```python
from build123d import *

# Parameters (mm, degrees)
BOSS_EXTRUDE1_DEPTH     = 10
SKETCH2_W               = 17.2
SKETCH2_H               = 43
CUT_EXTRUDE1_DEPTH      = 72.414284285
SKETCH3_W               = 90
SKETCH3_H               = 34
SKETCH3_W_2             = 80
SKETCH3_H_2             = 24
BOSS_EXTRUDE3_DEPTH     = 15
SKETCH4_W               = 49.6
SKETCH4_H               = 5
BOSS_EXTRUDE4_DEPTH     = 10
SKETCH5_W               = 15
SKETCH5_H               = 22
BOSS_EXTRUDE5_DEPTH     = 5
SKETCH6_W               = 90
SKETCH6_H               = 77
BOSS_EXTRUDE6_DEPTH     = 15
BOSS_EXTRUDE8_DEPTH     = 39
CHAMFER1_SIZE           = 64
CHAMFER1_SIZE_2         = 3.354097874
CHAMFER2_SIZE           = 64
CHAMFER2_SIZE_2         = 11.405813635
CHAMFER3_SIZE           = 64
CHAMFER3_SIZE_2         = 13.775745352
CUT_EXTRUDE3_DEPTH      = 95.500525601
CUT_EXTRUDE3_DEPTH_BACK = 95.500525601
SKETCH10_W              = 50
SKETCH10_H              = 27
SKETCH15_R              = 8
CUT_EXTRUDE5_DEPTH      = 122.227059686
CUT_EXTRUDE6_DEPTH      = 2.5
SKETCH18_W              = 29.6
SKETCH18_H              = 43
CUT_EXTRUDE7_DEPTH      = 10
CUT_EXTRUDE8_DEPTH      = 15
SKETCH21_W              = 29.6
SKETCH21_H              = 33
BOSS_EXTRUDE10_DEPTH    = 2.5
SKETCH23_W              = 2.05
SKETCH23_H              = 13
BOSS_EXTRUDE11_DEPTH    = 15
SKETCH24_OUTSIDE_W      = 133.046
SKETCH24_OUTSIDE_H      = 133.046
SKETCH24_OUTSIDE_W_2    = 90
SKETCH24_OUTSIDE_H_2    = 72
CUT_EXTRUDE10_DEPTH     = 61.5
SKETCH26_W              = 100
SKETCH26_H              = 100
CUT_EXTRUDE13_DEPTH     = 10


with BuildPart() as part:
    # Sketch1 → Boss-Extrude1 (new body)
    with BuildSketch(Plane(origin=(0, 0, 0), x_dir=(1, 0, 0), z_dir=(0, 1, 0))):
        with BuildLine():
            Line((-35, 50), (35, 50))
            ThreePointArc((35, 50), (45.606601718, 45.606601718), (50, 35))
            Line((50, 35), (50, -35))
            ThreePointArc((50, -35), (45.606601718, -45.606601718), (35, -50))
            Line((35, -50), (-35, -50))
            ThreePointArc((-35, -50), (-45.606601718, -45.606601718), (-50, -35))
            Line((-50, -35), (-50, 35))
            ThreePointArc((-50, 35), (-45.606601718, 45.606601718), (-35, 50))
        make_face()
    extrude(amount=BOSS_EXTRUDE1_DEPTH)

    # Sketch2 → Cut-Extrude1 (cut, through all)
    with BuildSketch(Plane(origin=(0, 10, 0), x_dir=(1, 0, 0), z_dir=(0, 1, 0))):
        with Locations((-33.4, 18.5)):
            Rectangle(SKETCH2_W, SKETCH2_H)
        with Locations((33.4, 18.5)):
            Rectangle(SKETCH2_W, SKETCH2_H)
    extrude(amount=-CUT_EXTRUDE1_DEPTH, mode=Mode.SUBTRACT)

    # Sketch3 → Boss-Extrude3 (add)
    with BuildSketch(Plane(origin=(0, 10, 0), x_dir=(1, 0, 0), z_dir=(0, 1, 0))):
        with Locations((0, -20)):
            Rectangle(SKETCH3_W, SKETCH3_H)
        with Locations((0, -20)):
            Rectangle(SKETCH3_W_2, SKETCH3_H_2, mode=Mode.SUBTRACT)
    extrude(amount=BOSS_EXTRUDE3_DEPTH)

    # Sketch4 → Boss-Extrude4 (add)
    with BuildSketch(Plane(origin=(0, 10, 0), x_dir=(1, 0, 0), z_dir=(0, 1, 0))):
        with Locations((0, 10)):
            Rectangle(SKETCH4_W, SKETCH4_H)
        with Locations((0, 27)):
            Rectangle(SKETCH4_W, SKETCH4_H)
    extrude(amount=BOSS_EXTRUDE4_DEPTH)

    # Sketch5 → Boss-Extrude5 (add)
    with BuildSketch(Plane(origin=(0, 20, 0), x_dir=(1, 0, 0), z_dir=(0, 1, 0))):
        with Locations((-17.3, 18.5)):
            Rectangle(SKETCH5_W, SKETCH5_H)
        with Locations((17.3, 18.5)):
            Rectangle(SKETCH5_W, SKETCH5_H)
    extrude(amount=BOSS_EXTRUDE5_DEPTH)

    # Sketch6 → Boss-Extrude6 (add)
    with BuildSketch(Plane(origin=(0, 10, 0), x_dir=(1, 0, 0), z_dir=(0, 1, 0))):
        with BuildLine():
            Line((-50, 35), (-50, -35))
            ThreePointArc((-50, -35), (-45.606601718, -45.606601718), (-35, -50))
            Line((-35, -50), (35, -50))
            ThreePointArc((35, -50), (45.606601718, -45.606601718), (50, -35))
            Line((50, -35), (50, 35))
            ThreePointArc((50, 35), (45.606601718, 45.606601718), (35, 50))
            Line((35, 50), (-35, 50))
            ThreePointArc((-35, 50), (-45.606601718, 45.606601718), (-50, 35))
        make_face()
        with Locations((0, 1.5)):
            Rectangle(SKETCH6_W, SKETCH6_H, mode=Mode.SUBTRACT)
    extrude(amount=BOSS_EXTRUDE6_DEPTH)

    # Sketch9 → Boss-Extrude8 (add)
    with BuildSketch(Plane(origin=(0, 25, 0), x_dir=(1, 0, 0), z_dir=(0, 1, 0))):
        with BuildLine():
            Line((-50, 35), (-50, -35))
            ThreePointArc((-50, -35), (-45.606601718, -45.606601718), (-35, -50))
            Line((-35, -50), (35, -50))
            ThreePointArc((35, -50), (45.606601718, -45.606601718), (50, -35))
            Line((50, -35), (50, 35))
            ThreePointArc((50, 35), (45.606601718, 45.606601718), (35, 50))
            Line((35, 50), (-35, 50))
            ThreePointArc((-35, 50), (-45.606601718, 45.606601718), (-50, 35))
        make_face()
        with BuildLine():
            Line((-45, 35), (-45, -32))
            Line((-45, -32), (45, -32))
            Line((45, -32), (45, 35))
            ThreePointArc((45, 35), (44.659258263, 37.588190451), (43.660254038, 40))
            Line((43.660254038, 40), (-43.660254038, 40))
            ThreePointArc((-43.660254038, 40), (-44.659258263, 37.588190451), (-45, 35))
        make_face(mode=Mode.SUBTRACT)
    extrude(amount=BOSS_EXTRUDE8_DEPTH)

    # Chamfer1
    # the kernel refuses this chamfer: 64, 3.354097874 mm, written as the material it takes off along each edge
    with BuildSketch(Plane(origin=(-35, 64, 50), x_dir=(0, -0.9999979738662979, 0.002013023422382214), z_dir=(1, 0, 0)), Plane(origin=(50, 64, 35), x_dir=(0.002013023422382214, -0.9999979738662979, 0), z_dir=(0, 0, -1)), Plane(origin=(-50, 64, -35), x_dir=(-0.002013023422382214, -0.9999979738662979, 0), z_dir=(0, 0, 1)), Plane(origin=(35, 64, -50), x_dir=(0, -0.9999979738662979, -0.002013023422382214), z_dir=(-1, 0, 0))) as chamfer1_piece_1:
        Polygon((CHAMFER1_SIZE * 0.999997973866, CHAMFER1_SIZE * 0.00201302342238), (-CHAMFER1_SIZE_2 * 0.00201302342245, CHAMFER1_SIZE_2 * 0.9999979739), (0, 0), align=None)
    extrude(amount=70, mode=Mode.SUBTRACT)
    with BuildSketch(Plane(origin=(35, 64, 35), x_dir=(0, 0, 1), z_dir=(-1, 0, 0))) as chamfer1_piece_2:
        Polygon((15, -CHAMFER1_SIZE), (15 - CHAMFER1_SIZE_2, 0), (15, 0), align=None)
    revolve(axis=Axis((35, 64, 35), (0, 1, 0)), revolution_arc=90, mode=Mode.SUBTRACT)
    with BuildSketch(Plane(origin=(-35, 64, 35), x_dir=(-1, 0, 0), z_dir=(0, 0, -1))) as chamfer1_piece_3:
        Polygon((15, -CHAMFER1_SIZE), (15 - CHAMFER1_SIZE_2, 0), (15, 0), align=None)
    revolve(axis=Axis((-35, 64, 35), (0, 1, 0)), revolution_arc=90, mode=Mode.SUBTRACT)
    with BuildSketch(Plane(origin=(35, 64, -35), x_dir=(1, 0, 0), z_dir=(0, 0, 1))) as chamfer1_piece_4:
        Polygon((15, -CHAMFER1_SIZE), (15 - CHAMFER1_SIZE_2, 0), (15, 0), align=None)
    revolve(axis=Axis((35, 64, -35), (0, 1, 0)), revolution_arc=90, mode=Mode.SUBTRACT)
    with BuildSketch(Plane(origin=(-35, 64, -35), x_dir=(0, 0, -1), z_dir=(1, 0, 0))) as chamfer1_piece_5:
        Polygon((15 - CHAMFER1_SIZE_2, 0), (15, -CHAMFER1_SIZE), (15, 0), align=None)
    revolve(axis=Axis((-35, 64, -35), (0, 1, 0)), revolution_arc=90, mode=Mode.SUBTRACT)

    # Chamfer2
    # the kernel refuses this chamfer: 64, 11.405813635 mm, written as the material it takes off along each edge
    with BuildSketch(Plane(origin=(201.306482971, 64, -46.645902126), x_dir=(0, -0.9982575003065525, -0.05900816114499234), z_dir=(-1, 0, 0))) as chamfer2_piece_1:
        Polygon((CHAMFER2_SIZE * 0.999977671636, CHAMFER2_SIZE * 0.0066825316561), (-CHAMFER2_SIZE_2 * 0.0590081611462, CHAMFER2_SIZE_2 * 0.998257500326), (0, 0), align=None)
    extrude(amount=402.612965942, mode=Mode.SUBTRACT)

    # Chamfer3
    # the kernel refuses this chamfer: 64, 13.775745352 mm, written as the material it takes off along each edge
    with BuildSketch(Plane(origin=(-201.265469314, 64, 46.645902126), x_dir=(0, -0.9981787050157903, 0.06032638604292662), z_dir=(1, 0, 0))) as chamfer3_piece_1:
        Polygon((CHAMFER3_SIZE * 0.999967974892, CHAMFER3_SIZE * 0.00800307379952), (-CHAMFER3_SIZE_2 * 0.060326386045, CHAMFER3_SIZE_2 * 0.99817870505), (0, 0), align=None)
    extrude(amount=402.530938629, mode=Mode.SUBTRACT)

    # Sketch10 → Cut-Extrude3 (cut, two sides: drawn at the far end of the back side and taken through both)
    with BuildSketch(Plane(origin=(0, 1.307501734, 0), x_dir=(0, 0, 1), z_dir=(-1, 0, 0)).offset(-CUT_EXTRUDE3_DEPTH_BACK)):
        with Locations((-22.129843227, 49.192498266)):
            Rectangle(SKETCH10_W, SKETCH10_H)
    extrude(amount=CUT_EXTRUDE3_DEPTH + CUT_EXTRUDE3_DEPTH_BACK, mode=Mode.SUBTRACT)

    # Sketch15 → Cut-Extrude5 (cut, through all)
    with BuildSketch(Plane.XY.offset(-40)):
        with Locations((-12.75, 20.25)):
            Circle(SKETCH15_R)
        with Locations((12.75, 20.25)):
            Circle(SKETCH15_R)
    extrude(amount=-CUT_EXTRUDE5_DEPTH, mode=Mode.SUBTRACT)

    # Sketch17 → Cut-Extrude6 (cut)
    with BuildSketch(Plane(origin=(0, 0, -29.5), x_dir=(-1, 0, 0), z_dir=(0, 0, -1))):
        Polygon((-24.8, 10), (24.8, 10), (24.8, 25), (9.8, 25), (9.8, 20), (-9.8, 20), (-9.8, 25), (-24.8, 25), align=None)
    extrude(amount=-CUT_EXTRUDE6_DEPTH, mode=Mode.SUBTRACT)

    # Sketch18 → Cut-Extrude7 (cut)
    with BuildSketch(Plane.XZ):
        with Locations((0, -18.5)):
            Rectangle(SKETCH18_W, SKETCH18_H)
    extrude(amount=-CUT_EXTRUDE7_DEPTH, mode=Mode.SUBTRACT)

    # Sketch20 → Cut-Extrude8 (cut)
    with BuildSketch(Plane.XZ.offset(-25)):
        with BuildLine():
            Line((-45, -35), (-45, -40))
            Line((-45, -40), (-43.660254038, -40))
            ThreePointArc((-43.660254038, -40), (-44.659258263, -37.588190451), (-45, -35))
        make_face()
        with BuildLine():
            Line((45, -40), (45, -35))
            ThreePointArc((45, -35), (44.659258263, -37.588190451), (43.660254038, -40))
            Line((43.660254038, -40), (45, -40))
        make_face()
    extrude(amount=-CUT_EXTRUDE8_DEPTH, mode=Mode.SUBTRACT)

    # Sketch21 → Boss-Extrude10 (add)
    with BuildSketch(Plane.XZ):
        with Locations((0, -13.5)):
            Rectangle(SKETCH21_W, SKETCH21_H)
    extrude(amount=-BOSS_EXTRUDE10_DEPTH)

    # Sketch23 → Boss-Extrude11 (add)
    with BuildSketch(Plane(origin=(0, 10, 0), x_dir=(1, 0, 0), z_dir=(0, 1, 0))):
        with Locations((-23.775, 33.5)):
            Rectangle(SKETCH23_W, SKETCH23_H)
        with Locations((23.775, 33.5)):
            Rectangle(SKETCH23_W, SKETCH23_H)
    extrude(amount=BOSS_EXTRUDE11_DEPTH)

    # Sketch24 outside → Cut-Extrude10 (cut)
    with BuildSketch(Plane(origin=(0, 64, 0), x_dir=(1, 0, 0), z_dir=(0, 1, 0))):
        Rectangle(SKETCH24_OUTSIDE_W, SKETCH24_OUTSIDE_H)
        with Locations((0, 4)):
            Rectangle(SKETCH24_OUTSIDE_W_2, SKETCH24_OUTSIDE_H_2, mode=Mode.SUBTRACT)
    extrude(amount=-CUT_EXTRUDE10_DEPTH, mode=Mode.SUBTRACT)

    # Sketch26 → Cut-Extrude13 (cut)
    with BuildSketch(Plane.XZ):
        Rectangle(SKETCH26_W, SKETCH26_H)
    extrude(amount=-CUT_EXTRUDE13_DEPTH, mode=Mode.SUBTRACT)


with BuildPart() as body_2:
    # of the pieces the cut leaves, the one that is kept (cut_extrude13_keep)
    add(part.part.solids().sort_by_distance((24.8, 25, -7.5))[0])


solid = body_2.part
```
For this review, take the finished solid that the model builds, in its own axes (mm). A direction names the side the tool comes from. Round coordinates to 2 decimals unless told otherwise and drop trailing zeros. Write each loop counter-clockwise with the first axis right and the second up, starting at its lowest first coordinate (ties: lowest second). Pieces come first, ordered by that corner, then holes. Notation, with made-up numbers: (31, 9.25) - (82, 9.25) arc R28 cw to (82, 38.25) - close; hole circle Ø11 at (45.25, 60.5). An arc over 180 degrees is marked (long way). Put each result on its own line as item: value.
Q1. Wall thickness on probe 1 along Z at (x, y) = (-21, 14.5); probe 2 along X at (y, z) = (14.25, -35); probe 3 along Z at (x, y) = (16.5, 21): over which ranges is each line inside the solid? List them lowest first.
Solved:
probe 1: z = -27 to -24.5, -12.5 to -7.5
probe 2: x = -24.8 to -22.75, 22.75 to 24.8
probe 3: z = -27 to -7.5
Q2. Mouldability with a two-part tool opening along Z and no side actions: class faces 4 (the face through (17, 20, -19)), 5 (the face through (24, 18, -40)), 6 (the face through (-17, 20, -19)), 7 (the face through (0, 20, -26)) as released by +Z, released by -Z, zero draft, split by the parting line, or undercut.
Solved:
face 4: undercut
face 5: released by -Z
face 6: undercut
face 7: zero draft
Q3. We need section D-D (z = -10). Give the boundary of the cut face in (x, y).
Solved:
outline: (-24.8, 10) - (24.8, 10) - (24.8, 25) - (9.8, 25) - (9.8, 20) - (-9.8, 20) - (-9.8, 25) - (-24.8, 25) - close
Q4. We need section A-A (z = -32). Give the boundary of the cut face in (x, y).
Solved:
outline: (-24.8, 10) - (-22.75, 10) - (-22.75, 25) - (-24.8, 25) - close; (22.75, 10) - (24.8, 10) - (24.8, 25) - (22.75, 25) - close
Q5. We need section C-C (x = -1). Give the boundary of the cut face in (y, z), and give its area (3 significant figures).
Solved:
outline: (10, -27) - (20, -27) - (20, -24.5) - (10, -24.5) - close; (10, -12.5) - (20, -12.5) - (20, -7.5) - (10, -7.5) - close
area: 75.0 mm2
Q6. Insertion check: pin 1 Ø6 at (x, z) = (-20, -18.5) entering from -Y; pin 2 Ø2 at (x, z) = (2.5, -26) entering from +Y; pin 3 Ø4.5 at (x, y) = (-1.5, 18.5) entering from -Z. Each pin has a flat end and moves straight along its axis. Give the tip position at first contact, or say it passes through.
Solved:
pin 1: stops at y = 20
pin 2: stops at y = 20
pin 3: stops at z = -27
Q7. We need section B-B (y = 21.5). Give the boundary of the cut face in (x, z), and give its area (3 significant figures).
Solved:
outline: (-24.8, -40) - (-22.75, -40) - (-22.75, -27) - (-9.8, -27) - (-9.8, -7.5) - (-24.8, -7.5) - close; (9.8, -27) - (22.75, -27) - (22.75, -40) - (24.8, -40) - (24.8, -7.5) - (9.8, -7.5) - close
area: 638 mm2
Q8. Machinability: for faces 1 (the face through (0, 15, -24.5)), 2 (the face through (0, 20, -10)), 3 (the face through (22.75, 17, -33)), which of the approach directions +Z, -Z, +X, -X, +Y, -Y give a long, thin tool a straight path to every point of the face, cutting with its end or side? Answer none if there is none.
Solved:
face 1: +X, -X, -Y
face 2: +Z, -Z, +Y
face 3: -Z, +Y, -Y
